Work out the finished part from the listing and answer in its coordinate system (mm). A direction names the side the tool comes from. Coordinates: 2 decimals unless noted, no trailing zeros. Loops run counter-clockwise (first coordinate to the right, second up) from the corner with the lowest first, then second, coordinate; pieces in that order, holes last. Notation, with made-up numbers: (54.25, -14) - (97.25, -14) arc R28 cw to (97.25, 16) - close; hole circle Ø4 at (71, 69.5). An arc over 180 degrees is marked (long way). Write each question's results on one line, items separated by ' | '. Start each with the question number.
1. A cutting plane is placed at A-A on y = 0. Determine the outline of the cut face in (x, z), then the cut area to 3 significant figures.
2. Each of these flat-tipped pins is pushed along its axis until it touches: P1, Ø10, axis at x = 41, z = -509, coming from the +Y side; P2, Ø1.5, axis at x = -40.5, z = -2269, coming from the -Y side; P3, Ø1.5, axis at x = -86.5, z = -311, coming from the -Y side. Where does it stop, or does it pass through?
3. Determine the mould class of faces 5 (the cylindrical face through (-22.025, -99.184, -1280.025)), 6 (the cylindrical face through (-22.025, 99.184, 56.883)), 7 (the flat face through (-10, -103, -2634.5)) for opening direction Z: released by +Z, released by -Z, zero draft, split by the parting line, or undercut.
4. A cutting plane is placed at C-C on z = -1467. Determine the outline of the cut face in (x, y), then the cut area to 3 significant figures.
5. Which of the six approach directions +Z, -Z, +X, -X, +Y, -Y give full straight-line access (tool end or side, diameter ignored) to faces 1 (the flat face through (-1, 1, 76.2)), 2 (the flat face through (10, -103, 38.1)), 3 (the cylindrical face through (22.025, 99.184, -2653.283)), 4 (the flat face through (-10, -103, -2596.4))?
6. Find the intervals of material crossed by line 1 along Z through (x, y) = (76, 91); line 2 along Y through (x, z) = (-7, -2038.5); line 3 along X through (y, z) = (31, -1178), in increasing order. Write a range as [from, to].
Autodesk Inventor part; units mm, degrees
ref_plane "YZ Plane" through (0, 0, 0) normal (1, 0, 0) x (0, 1, 0)
ref_plane "XZ Plane" through (0, 0, 0) normal (0, 1, 0) x (-1, 0, 0)
ref_plane "XY Plane" through (0, 0, 0) normal (0, 0, 1) x (1, 0, 0)
sketch "Sketch1" plane through (0, 0, 0) normal (0, 0, 1) x (1, 0, 0)
  circle A0 centre (0, 0) radius 101.6
  dimension "d0" = 203.2
extrude "Extrusion1" add sketch "Sketch1" against normal blind 2596.4
sketch "Sketch2" plane through (0, 0, 0) normal (0, 0, 1) x (1, 0, 0)
  circle A0 centre (0, 0) radius 139.7
  dimension "d3" = 279.4
extrude "Extrusion2" add sketch "Sketch2" along normal blind 38.1
sketch "Sketch3" plane through (0, 0, -2596.4) normal (0, 0, -1) x (-1, 0, 0)
  circle A0 centre (0, 0) radius 139.7
extrude "Extrusion3" add sketch "Sketch3" along normal blind 38.1
sketch "Sketch4" plane through (0, 0, 38.1) normal (0, 0, 1) x (1, 0, 0)
  circle A0 centre (0, 0) radius 101.6
extrude "Extrusion4" add sketch "Sketch4" along normal blind 38.1
sketch "Sketch5" plane through (0, 0, -2634.5) normal (0, 0, -1) x (-1, 0, 0)
  circle A0 centre (0, 0) radius 101.6
extrude "Extrusion5" add sketch "Sketch5" along normal blind 38.1
properties part number "dry_pipe_new"
Values:
1) outline: (-139.7, -2634.5) - (-101.6, -2634.5) - (-101.6, -2672.6) - (101.6, -2672.6) - (101.6, -2634.5) - (139.7, -2634.5) - (139.7, -2596.4) - (101.6, -2596.4) - (101.6, 0) - (139.7, 0) - (139.7, 38.1) - (101.6, 38.1) - (101.6, 76.2) - (-101.6, 76.2) - (-101.6, 38.1) - (-139.7, 38.1) - (-139.7, 0) - (-101.6, 0) - (-101.6, -2596.4) - (-139.7, -2596.4) - close | area: 564,000 mm^2
2) P1: y = 95.01 | P2: y = -93.5 | P3: y = -54.49
3) face 5: undercut | face 6: zero draft | face 7: released by -Z
4) outline: circle Ø203.2 at (0, 0) | area: 32,400 mm^2
5) face 1: +Z, +X, -X, +Y, -Y | face 2: +Z | face 3: -Z | face 4: none
6) line 1: [-2634.5, -2596.4], [0, 38.1] | line 2: [-101.36, 101.36] | line 3: [-96.76, 96.76]
